The model under review builds one solid part; all positions refer to its coordinate system, in mm. A direction names the side the tool comes from. Give positions to 0.01 mm unless a question says otherwise; leave off trailing zeros. Loops run counter-clockwise (first coordinate to the right, second up) from the corner with the lowest first, then second, coordinate; pieces in that order, holes last. Notation, with made-up numbers: (81.5, -37.75) -> (85.5, -37.75) arc R21 cw to (85.5, -17.75) -> close; hole circle Ø8 at (73, 10.25). An arc over 180 degrees is marked (long way). Write each question's results on one line, items separated by ' | '. Start each with the question number.
Q1. We need section C-C (y = 12). Write out the cut boundary in (x, z), plus the area to 3 significant figures.
Q2. Mouldability with a two-part tool opening along X and no side actions: class faces 1 (the face through (-21.215, -16.199, 16.731)), 2 (the face through (20, 0, 18)), 3 (the face through (-2, -16, 33)) as released by +X, released by -X, zero draft, split by the parting line, or undercut.
Q3. Insertion check: pin 1 Ø15 at (x, y) = (9.5, -7) entering from +Z. The pin has a flat end and moves straight along its axis. Give the tip position at first contact, or say it passes through.
Q4. Wall thickness on L1, parallel to X at y = -12, z = 7; L2, parallel to Y at x = -7, z = 21.5; L3, parallel to Z at x = -10.5, y = 12: over which ranges is each line inside the solid? List them lowest first. Write a range as [from, to].
Q5. We need section B-B (x = 6). Write out the cut boundary in (y, z).
Q6. We need section A-A (z = 16). Write out the cut boundary in (x, y), plus the area to 3 significant figures.
Q7. Machinability: for faces 4 (the face through (19.715, 14.699, 17.79)), 5 (the face through (21.5, 0, 16)), which of the approach directions +Z, -Z, +X, -X, +Y, -Y give a long, thin tool a straight path to every point of the face, cutting with its end or side? Answer none if there is none.
from build123d import *

# Parameters (mm, degrees)
F0_W     = 43
F0_H     = 33
F1_DEPTH = 33
F2_W     = 40
F2_H     = 30
F3_DEPTH = 30
F4_R     = 1
F5_R     = 1


with BuildPart() as f1:
    # F0 (on Top) → F1 (new body)
    with BuildSketch(Plane.XY):
        Rectangle(F0_W, F0_H)
    extrude(amount=F1_DEPTH)

    # F2 (on face) → F3 (cut)
    with BuildSketch(Plane.XY.offset(33)):
        Rectangle(F2_W, F2_H)
    extrude(amount=-F3_DEPTH, mode=Mode.SUBTRACT)

    # F4
    f4_edges = [f1.edges().sort_by_distance(p)[0] for p in [
        (-21.5, -16.5, 16.5),
        (21.5, -16.5, 16.5),
        (21.5, 16.5, 16.5),
        (-21.5, 16.5, 16.5),
    ]]
    fillet(f4_edges, radius=F4_R)

    # F5
    f5_edges = [f1.edges().sort_by_distance(p)[0] for p in [
        (-20, -15, 18),
        (-20, 15, 18),
        (20, 15, 18),
        (20, -15, 18),
    ]]
    fillet(f5_edges, radius=F5_R)


solid = f1.part
Output:
1) outline: (-21.5, 0) -> (21.5, 0) -> (21.5, 33) -> (20, 33) -> (20, 3) -> (-20, 3) -> (-20, 33) -> (-21.5, 33) -> close | area: 219 mm2
2) face 1: released by -X | face 2: undercut | face 3: zero draft
3) pin 1: z = 3
4) L1: [-21.5, -20], [20, 21.5] | L2: [-16.5, -15], [15, 16.5] | L3: [0, 3]
5) outline: (-16.5, 0) -> (16.5, 0) -> (16.5, 33) -> (15, 33) -> (15, 3) -> (-15, 3) -> (-15, 33) -> (-16.5, 33) -> close
6) outline: (-21.5, -15.5) arc R1 ccw to (-20.5, -16.5) -> (20.5, -16.5) arc R1 ccw to (21.5, -15.5) -> (21.5, 15.5) arc R1 ccw to (20.5, 16.5) -> (-20.5, 16.5) arc R1 ccw to (-21.5, 15.5) -> close; hole (-20, -14) arc R1 ccw to (-19, -15) -> (19, -15) arc R1 ccw to (20, -14) -> (20, 14) arc R1 ccw to (19, 15) -> (-19, 15) arc R1 ccw to (-20, 14) -> close | area: 219 mm2
7) face 4: +Z | face 5: +Z, -Z, +X, +Y, -Y
